Input: part model. Units: mm. Frame: model coordinates. Coordinates: 2 decimals unless noted, no trailing zeros. Write each loop counter-clockwise with the first axis right and the second up, starting at its lowest first coordinate (ties: lowest second). Pieces come first, ordered by that corner, then holes. Notation, with made-up numbers: (63, -34.75) - (88, -34.75) arc R33 cw to (88, 4.25) - close; hole circle Ø10 at (34, -8). An arc over 180 degrees is marked (long way). Put each result on its own line as item: value. Start each with the question number.
1. Line query: line 1 (Y direction, x = -1.2, z = -11.25); line 2 (Y direction, x = 0.8, z = -11.75); line 3 (X direction, y = 2.45, z = -7.5). Output: solid intervals per line, ascending.
2. Pin query (flat end, axial travel): pin 1 (1 mm diameter, centred on x = 2.5, z = -8.5, fed in from +Y). Return the tip coordinate at first contact, or that it passes through.
3. Cut plane A-A, the plane z = -1.5. Return loops of the section in (x, y).
from build123d import *

# Parameters (mm, degrees)
SKETCH2_R           = 3
BOSS_EXTRUDE1_DEPTH = 15.5
SKETCH5_R           = 2.75
BOSS_EXTRUDE2_DEPTH = 0.25
FILLET3_R           = 0.75
SKETCH6_R           = 2.75
BOSS_EXTRUDE3_DEPTH = 0.25
FILLET4_R           = 0.75


with BuildPart() as part:
    # Sketch2 → Boss-Extrude1 (new body)
    with BuildSketch(Plane.XY):
        Circle(SKETCH2_R)
    extrude(amount=-BOSS_EXTRUDE1_DEPTH)

    # Sketch5 → Boss-Extrude2 (add)
    with BuildSketch(Plane.XY):
        Circle(SKETCH5_R)
    extrude(amount=BOSS_EXTRUDE2_DEPTH)

    # Fillet3
    # the kernel refuses this fillet: 0.75 mm, written as the material it takes off along each edge
    with BuildSketch(Plane(origin=(0, 0, 0), x_dir=(1, 0, 0), z_dir=(0, -1, 0))) as fillet3_piece_1:
        with BuildLine():
            CenterArc((2.25, -0.559016994), FILLET3_R, 0, 48.189685104)
            Line((2.75, 0), (2.76, 0.01118034))
            ThreePointArc((2.76, 0.01118034), (2.875, 0.015), (3, 0.015))
            Line((3, 0.015), (3.015, 0))
            Line((3.015, 0), (3.015, -0.559016994))
            Line((3.015, -0.559016994), (3, -0.559016994))
        make_face()
    revolve(axis=Axis((0, 0, 0), (0, 0, 1)), mode=Mode.SUBTRACT)
    with BuildSketch(Plane(origin=(0, 0, 0.25), x_dir=(1, 0, 0), z_dir=(0, -1, 0))) as fillet3_piece_2:
        with BuildLine():
            CenterArc((2.190983006, -0.75), FILLET3_R, 41.810314896, 48.189685104)
            Line((2.190983006, 0), (2.190983006, 0.015))
            Line((2.190983006, 0.015), (2.75, 0.015))
            Line((2.75, 0.015), (2.765, 0))
            ThreePointArc((2.765, 0), (2.765, -0.125), (2.76118034, -0.24))
            Line((2.76118034, -0.24), (2.75, -0.25))
        make_face()
    revolve(axis=Axis((0, 0, 0.25), (0, 0, 1)), mode=Mode.SUBTRACT)

    # Sketch6 → Boss-Extrude3 (add)
    with BuildSketch(Plane(origin=(0, 0, -15.5), x_dir=(-1, 0, 0), z_dir=(0, 0, -1))):
        Circle(SKETCH6_R)
    extrude(amount=BOSS_EXTRUDE3_DEPTH)

    # Fillet4
    # the kernel refuses this fillet: 0.75 mm, written as the material it takes off along each edge
    with BuildSketch(Plane(origin=(0, 0, -15.75), x_dir=(-1, 0, 0), z_dir=(0, -1, 0))) as fillet4_piece_1:
        with BuildLine():
            CenterArc((2.190983006, -0.75), FILLET4_R, 41.810314896, 48.189685104)
            Line((2.190983006, 0), (2.190983006, 0.015))
            Line((2.190983006, 0.015), (2.75, 0.015))
            Line((2.75, 0.015), (2.765, 0))
            ThreePointArc((2.765, 0), (2.765, -0.125), (2.76118034, -0.24))
            Line((2.76118034, -0.24), (2.75, -0.25))
        make_face()
    revolve(axis=Axis((0, 0, -15.75), (0, 0, -1)), mode=Mode.SUBTRACT)
    with BuildSketch(Plane(origin=(0, 0, -15.5), x_dir=(1, 0, 0), z_dir=(0, -1, 0))) as fillet4_piece_2:
        with BuildLine():
            CenterArc((2.25, 0.559016994), FILLET4_R, 311.810314896, 48.189685104)
            Line((2.75, 0), (2.76, -0.01118034))
            ThreePointArc((2.76, -0.01118034), (2.875, -0.015), (3, -0.015))
            Line((3, -0.015), (3.015, 0))
            Line((3.015, 0), (3.015, 0.559016994))
            Line((3.015, 0.559016994), (3, 0.559016994))
        make_face()
    revolve(axis=Axis((0, 0, -15.5), (0, 0, 1)), mode=Mode.SUBTRACT)


solid = part.part
Report:
1. line 1: y = -2.75 to 2.75
1. line 2: y = -2.89 to 2.89
1. line 3: x = -1.73 to 1.73
2. pin 1: stops at y = 2.24
3. outline: circle Ø6 at (0, 0)
